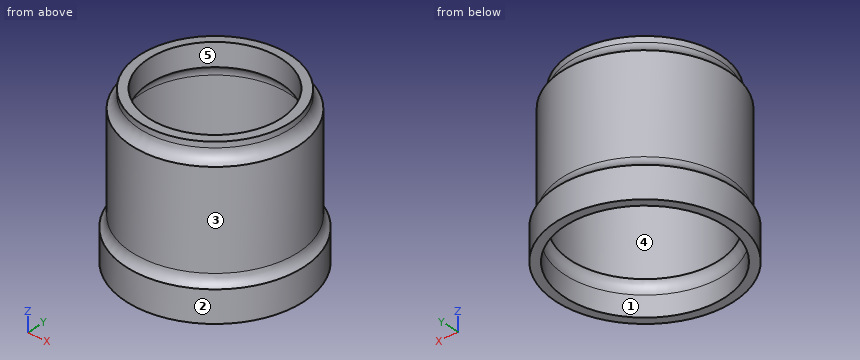
from build123d import *


# Not quite as in the source:
# - a fillet or chamfer that OpenCascade refuses, or shapes differently, is made with other operations: its cross-section is extruded or revolved along the edge and cut away or added


with BuildPart() as f1:
    # F0 (on Front) → F1 (revolve)
    with BuildSketch(Plane.XZ):
        Polygon((-16.5, 0), (-16.5, 5.7386059155), (-14.75, 5.7386059155), (-14.75, 10.8408229426), (-16.75, 10.7678563523), (-16.75, 6.7678563523), (-18.5, 6.7678563523), (-18.5, -17.2321436477), (-19.75, -17.2321436477), (-19.75, -24.2321436477), (-17.75, -24.2321436477), (-17.75, -17.2321436477), (-16.5, -17.2300804406), align=None)
    revolve(axis=Axis((0, 0, -1.1706372043), (0, 0, -1)))

    # F2: fillet of radius 3 on 4 edges, made by hand

    # F2_s1 → F2_t2 (revolve)
    with BuildSketch(Plane.XZ):
        with BuildLine():
            ThreePointArc((-18.5, 6.7678563523), (-17.2251237654, 7.8748492064), (-16.75, 9.495034381))
            Line((-16.75, 9.495034381), (-16.75, 6.7678563523))
            Line((-16.75, 6.7678563523), (-18.5, 6.7678563523))
        make_face()
    revolve(axis=Axis((0, 0, 6.7678563523), (0, 0, -1)))

    # F2_s3 → F2_t4 (revolve)
    with BuildSketch(Plane.XZ):
        with BuildLine():
            ThreePointArc((-19.75, -17.2321436477), (-18.830730437, -16.1647514552), (-18.5, -14.7954450615))
            Line((-18.5, -14.7954450615), (-18.5, -17.2321436477))
            Line((-18.5, -17.2321436477), (-19.75, -17.2321436477))
        make_face()
    revolve(axis=Axis((0, 0, -17.2321436477), (0, 0, -1)))

    # F2_s5 → F2_t6 (revolve)
    with BuildSketch(Plane.XZ):
        with BuildLine():
            ThreePointArc((-16.5, -17.2300804406), (-17.419269563, -18.2974726331), (-17.75, -19.6667790268))
            Line((-17.75, -19.6667790268), (-17.75, -17.2321436477))
            Line((-17.75, -17.2321436477), (-16.5, -17.2300804406))
        make_face()
    revolve(axis=Axis((0, 0, -17.2321436477), (0, 0, -1)))

    # F2_s7 → F2_t8 (revolve)
    with BuildSketch(Plane.XZ):
        with BuildLine():
            ThreePointArc((-16.5, 3.0114278869), (-16.0248762346, 4.6316130615), (-14.75, 5.7386059155))
            Line((-14.75, 5.7386059155), (-16.5, 5.7386059155))
            Line((-16.5, 5.7386059155), (-16.5, 3.0114278869))
        make_face()
    revolve(axis=Axis((0, 0, 5.7386059155), (0, 0, -1)))


solid = f1.part
Part model, mm, in its own coordinate system. Face numbers are marked on the shaded views. A direction names the side the tool comes from. Coordinates: 2 decimals unless noted, no trailing zeros. Order: outer loops, then holes, each group sorted by start corner. A loop starts at its lowest first (then second) coordinate and runs counter-clockwise, first axis right, second up. Notation, with made-up numbers: (66, 49.5) - (97, 49.5) arc R23 cw to (97, 87.5) - close; hole circle Ø6 at (83, 22). An arc over 180 degrees is marked (long way). Use CSV: the item, a comma, the result in double quotes.
Item 1: Saw through at D-D on z = -19. Give the cut face in (x, y), and give its area (3 significant figures).
Solved:
outline,"circle Ø39.5 at (0, 0); hole circle Ø35.35 at (0, 0)"
area,"244 mm²"
Item 2: Probe probe 1 along Y at (x, z) = (0, -11.75); probe 2 along Y at (x, z) = (0, -23.2); probe 3 along X at (y, z) = (14.5, -21.5). List the from-to ranges inside material, lowest first.
Solved:
probe 1,"y = -18.5 to -16.5, 16.5 to 18.5"
probe 2,"y = -19.75 to -17.75, 17.75 to 19.75"
probe 3,"x = -13.41 to -10.24, 10.24 to 13.41"
Item 3: Drop flat-ended pins along their axis: P1, Ø3, axis at x = -12, y = -4.5, coming from the -Z side; P2, Ø6, axis at y = 0, z = -8.5, coming from the +X side; P3, Ø10, axis at x = -7, z = -5, coming from the -Y side; P4, Ø12, axis at y = -11.5, z = -4, coming from the +X side. Give the stop position or say it passes through.
Solved:
P1,"passes through"
P2,"stops at x = 18.5"
P3,"stops at y = -18.39"
P4,"stops at x = 17.66"
Item 4: 3-axis set-ups, long thin cutter, end or side, ignore diameter. For the marked faces 3, 4 and 5: which of +Z, -Z, +X, -X, +Y, -Y reach the whole face in a straight line?
Solved:
face 3,"+Z"
face 4,"-Z"
face 5,"+Z, -Z"
Item 5: Saw through at A-A on y = 0. Give the cut face in (x, z), and give its area (3 significant figures).
Solved:
outline,"(-19.75, -24.23) - (-17.75, -24.23) - (-17.75, -19.67) arc R3 cw to (-16.5, -17.23) - (-16.5, 3.01) arc R3 cw to (-14.75, 5.74) - (-14.75, 10.84) - (-16.75, 10.77) - (-16.75, 9.5) arc R3 cw to (-18.5, 6.77) - (-18.5, -14.8) arc R3 cw to (-19.75, -17.23) - close; (14.75, 5.74) arc R3 cw to (16.5, 3.01) - (16.5, -17.23) arc R3 cw to (17.75, -19.67) - (17.75, -24.23) - (19.75, -24.23) - (19.75, -17.23) arc R3 cw to (18.5, -14.8) - (18.5, 6.77) arc R3 cw to (16.75, 9.5) - (16.75, 10.77) - (14.75, 10.84) - close"
area,"153 mm²"
Item 6: Saw through at C-C on z = -7. Give the cut face in (x, y), and give its area (3 significant figures).
Solved:
outline,"circle Ø37 at (0, 0); hole circle Ø33 at (0, 0)"
area,"220 mm²"
Item 7: Mould opens along Y. For the marked faces 1 and 2 say: +Y half, -Y half, draft (parallel to the pull), parting line (faces both ways), or undercut.
Solved:
face 1,"undercut"
face 2,"parting line"
